Work out the finished part from the listing and answer in its coordinate system (mm). A direction names the side the tool comes from. Give positions to 0.01 mm unless a question says otherwise; leave off trailing zeros. Loops run counter-clockwise (first coordinate to the right, second up) from the corner with the lowest first, then second, coordinate; pieces in that order, holes last. Notation, with made-up numbers: M 80,-26 L 125,-26 A7 cw 125,-15 Z; hole C -11.5,86 d4. An arc over 180 degrees is marked long. Write item = value, one per line. Start each with the question number.
1. Section C-C on z = 3.25 is taken. Give the number of separate pieces and of enclosed holes in the cut face, plus the area to 3 significant figures.
2. Flat-ended cylindrical pins translate along their axes: pin 1 Ø2.5 at (y, z) = (6.5, 3) entering from -X; pin 2 Ø1.5 at (y, z) = (4.5, 1) entering from -X. Find the tip coordinate at first contact, or state that the pin passes through.
3. Consider L1, parallel to Y at x = 7.5, z = 1.6; L2, parallel to Y at x = 47.5, z = 1.75; L3, parallel to Y at x = 30.54, z = 3.75. Determine where each line is inside the solid, lowest interval first. Write a range as [from, to].
4. Section A-A on x = 64.46 is taken. Determine the outline of the cut face in (y, z).
5. Section B-B on y = 15 is taken. Determine the outline of the cut face in (x, z), plus the area to 3 significant figures.
6. The mould has two halves that part along X. Classify faces 1 (the face through (2.281, 2.406, 2.465)), 2 (the face through (48, 30, 2)), 3 (the face through (87, 25, 2)): released by +X, released by -X, zero draft, split by the parting line, or undercut.
7. For faces 4 (the face through (92.719, 27.594, 2.465)), 5 (the face through (7, 25, 2)), determine the directions among +Z, -Z, +X, -X, +Y, -Y from which every point of the face is accessible in a straight line to the end or side of a thin tool.
8. Section D-D on x = 47.5 is taken. Determine the outline of the cut face in (y, z).
```python
from build123d import *

# Parameters (mm, degrees)
ESQUISSE1_R        = 1.5
ESQUISSE1_R_2      = 2
ESQUISSE1_R_3      = 2.5
ESQUISSE1_W        = 5
ESQUISSE1_H        = 5
BOSS_EXTRU_1_DEPTH = 5


with BuildPart() as part:
    # Esquisse1 → Boss.-Extru.1 (new body)
    with BuildSketch(Plane.XY):
        with BuildLine():
            Line((8, 0), (87, 0))
            ThreePointArc((87, 0), (92.656854249, 2.343145751), (95, 8))
            Line((95, 8), (95, 22))
            ThreePointArc((95, 22), (92.656854249, 27.656854249), (87, 30))
            Line((87, 30), (8, 30))
            ThreePointArc((8, 30), (2.343145751, 27.656854249), (0, 22))
            Line((0, 22), (0, 8))
            ThreePointArc((0, 8), (2.343145751, 2.343145751), (8, 0))
        make_face()
        with Locations((7.5, 15)):
            Circle(ESQUISSE1_R, mode=Mode.SUBTRACT)
        with Locations((87.5, 15)):
            Circle(ESQUISSE1_R, mode=Mode.SUBTRACT)
        with Locations((30.54, 15)):
            Circle(ESQUISSE1_R_2, mode=Mode.SUBTRACT)
        with Locations((64.46, 15)):
            Circle(ESQUISSE1_R_2, mode=Mode.SUBTRACT)
        with Locations((47.5, 15)):
            Circle(ESQUISSE1_R_3, mode=Mode.SUBTRACT)
        with Locations((7.5, 22.5)):
            Rectangle(ESQUISSE1_W, ESQUISSE1_H, mode=Mode.SUBTRACT)
        with Locations((87.5, 22.5)):
            Rectangle(ESQUISSE1_W, ESQUISSE1_H, mode=Mode.SUBTRACT)
        with Locations((87.5, 7.5)):
            Rectangle(ESQUISSE1_W, ESQUISSE1_H, mode=Mode.SUBTRACT)
        with Locations((7.5, 7.5)):
            Rectangle(ESQUISSE1_W, ESQUISSE1_H, mode=Mode.SUBTRACT)
    extrude(amount=BOSS_EXTRU_1_DEPTH)


solid = part.part
```
Verdict:
q1.separate_pieces = 1
q1.enclosed_holes = 9
q1.area = 2,640 mm2
q2.pin_1 = 0
q2.pin_2 = 0.49
q3.L1 = [0.02, 5], [10, 13.5], [16.5, 20], [25, 29.98]
q3.L2 = [0, 12.5], [17.5, 30]
q3.L3 = [0, 13], [17, 30]
q4.outline = M 0,0 L 13,0 L 13,5 L 0,5 Z; M 17,0 L 30,0 L 30,5 L 17,5 Z
q5.outline = M 0,0 L 6,0 L 6,5 L 0,5 Z; M 9,0 L 28.54,0 L 28.54,5 L 9,5 Z; M 32.54,0 L 45,0 L 45,5 L 32.54,5 Z; M 50,0 L 62.46,0 L 62.46,5 L 50,5 Z; M 66.46,0 L 86,0 L 86,5 L 66.46,5 Z; M 89,0 L 95,0 L 95,5 L 89,5 Z
q5.area = 380 mm2
q6.face_1 = released by -X
q6.face_2 = zero draft
q6.face_3 = undercut
q7.face_4 = +Z, -Z, +X, +Y
q7.face_5 = +Z, -Z
q8.outline = M 0,0 L 12.5,0 L 12.5,5 L 0,5 Z; M 17.5,0 L 30,0 L 30,5 L 17.5,5 Z
